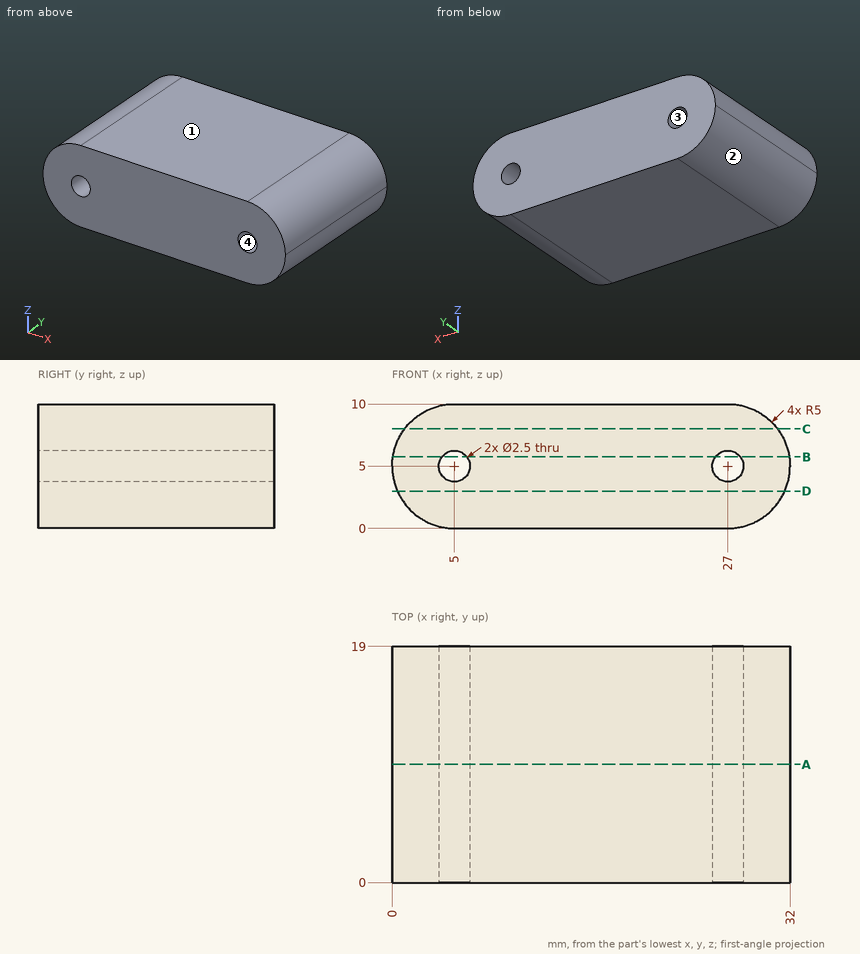
Geometry: see drawing. Coordinates: mm, zero at the bounding-box minimum. Coordinates: 2 decimals unless noted, no trailing zeros. Loops run counter-clockwise (first coordinate to the right, second up) from the corner with the lowest first, then second, coordinate; pieces in that order, holes last. Notation, with made-up numbers: (30.5, 9.5) - (46.5, 9.5) arc R17 ccw to (46.5, 23.5) - close; hole circle Ø7 at (-24, 33.5). An arc over 180 degrees is marked (long way). Return JSON: item names as keys, results as strings.
Q1. Section B-B, the plane z = 5.75. Return loops of the section in (x, y), plus the area to 3 significant figures.
Results:
{"outline": "(0.06, 0) - (4, 0) - (4, 19) - (0.06, 19) - close; (6, 0) - (26, 0) - (26, 19) - (6, 19) - close; (28, 0) - (31.94, 0) - (31.94, 19) - (28, 19) - close", "area": "530 mm2"}
Q2. Section D-D, the plane z = 3. Return loops of the section in (x, y), plus the area to 3 significant figures.
Results:
{"outline": "(0.42, 0) - (31.58, 0) - (31.58, 19) - (0.42, 19) - close", "area": "592 mm2"}
Q3. Contact query for a flat-ended pin moving along its axis: P1, Ø1, axis at y = 2.5, z = 8, coming from the -X side. Output: stop coordinate, or through.
Results:
{"P1": "x = 0.67"}
Q4. Section C-C, the plane z = 8. Return loops of the section in (x, y), plus the area to 3 significant figures.
Results:
{"outline": "(1, 0) - (31, 0) - (31, 19) - (1, 19) - close", "area": "570 mm2"}
Q5. Mould query, pull axis X, two halves, no side actions, for the marked faces 1, 2, 3 and 4. Classes: released by +X, released by -X, zero draft, split by the parting line, or undercut.
Results:
{"face 1": "zero draft", "face 2": "released by -X", "face 3": "undercut", "face 4": "undercut"}
Q6. Section A-A, the plane y = 9.5. Give the number of separate pieces and of enclosed holes in the cut face, plus the area to 3 significant figures.
Results:
{"separate pieces": "1", "enclosed holes": "2", "area": "289 mm2"}
Q7. Material intervals for line 1 along X through (y, z) = (5.25, 5); line 2 along X through (y, z) = (3.75, 6); line 3 along Z through (x, y) = (5.5, 10.5), sorted ascending.
Results:
{"line 1": "0 to 3.75, 6.25 to 25.75, 28.25 to 32", "line 2": "0.1 to 4.25, 5.75 to 26.25, 27.75 to 31.9", "line 3": "0 to 3.85, 6.15 to 10"}
